Input: part model. Units: mm. Frame: model coordinates. A direction names the side the tool comes from. Coordinates: 2 decimals unless noted, no trailing zeros. Loops run counter-clockwise (first coordinate to the right, second up) from the corner with the lowest first, then second, coordinate; pieces in that order, holes last. Notation, with made-up numbers: (57, 67.25) -> (89, 67.25) arc R27 cw to (89, 87.25) -> close; hole circle Ø2 at (58, 77.5). An arc over 180 degrees is marked (long way). Put each result on its own line as item: value. Start each with the question number.
1) Cut plane B-B (z = -0.5). Return the cut outline in (x, y).
2) Cut plane A-A (z = 3). State how many separate pieces and enclosed holes the cut face has, plus the area to 3 significant figures.
3) Pull-direction query (X, two-part tool) for faces 1 (the flat face through (0, -2, 5.5)), 2 (the cylindrical face through (2.92, -14.18, 5.88)), 3 (the cylindrical face through (17.856, 3.771, 4.277)), 4 (the flat face through (0, 0, 6.5)); classes: pulls with the +X half, pulls with the -X half, needs draft (parallel to the pull), parting line crosses it, or undercut.
4) Set-up query: faces 5 (the cylindrical face through (1.269, 9.667, 2.712)), 6 (the cylindrical face through (8.19, 16.31, 4.28)), 7 (the cylindrical face through (1.03, -14.47, 5.48)). Return all of +Z, -Z, +X, -X, +Y, -Y with unobstructed straight access to the full face (end or side cutting, diameter ignored); none if empty.
5) Material intervals for L1, parallel to Y at x = 0, z = 1.1; L2, parallel to Z at x = -9, y = 1.5; L3, parallel to X at y = -4.5, z = 4, sorted ascending.
6) Contact query for flat-ended pins moving along their axis: P1, Ø8, axis at x = 7, y = 10, coming from the -Z side; P2, Ø4, axis at x = -3.5, z = 3, coming from the -Y side; P3, Ø4, axis at x = 13, z = 2.5, coming from the -Y side; P4, Ø6.5, axis at x = -1, y = 0, coming from the -Z side. Output: stop coordinate, or through.
from build123d import *

# Parameters (mm, degrees)
SKETCH_1_R               = 11
EXTRUDE_1_DEPTH          = 6.5
SKETCH_2_R               = 9.75
CUT_EXTRUDE_1_DEPTH      = 5.5
SKETCH_3_R               = 0.7
EXTRUDE_2_DEPTH          = 7.5
CHAMFER_1_SIZE           = 0.6
EXTRUDE_START            = -10
EXTRUDE_3_DEPTH          = 23
PATTERN_CIRCULAR_1_COUNT = 7
FILLET_1_R               = 0.3
SKETCH_5_OUTSIDE_W       = 86.532
SKETCH_5_OUTSIDE_H       = 84.877
SKETCH_5_OUTSIDE_R       = 18.25
CUT_EXTRUDE_2_DEPTH      = 23


with BuildPart() as part:
    # Sketch 1 → Extrude 1 (new body)
    with BuildSketch(Plane.XY):
        Circle(SKETCH_1_R)
    extrude(amount=EXTRUDE_1_DEPTH)

    # Sketch 2 → Cut-Extrude 1 (cut)
    with BuildSketch(Plane(origin=(0, 0, 0), x_dir=(-1, 0, 0), z_dir=(0, 0, -1))):
        Circle(SKETCH_2_R)
    extrude(amount=-CUT_EXTRUDE_1_DEPTH, mode=Mode.SUBTRACT)

    # Sketch 3 → Extrude 2 (add)
    with BuildSketch(Plane(origin=(0, 0, 5.5), x_dir=(-1, 0, 0), z_dir=(0, 0, -1))):
        Circle(SKETCH_3_R)
    extrude(amount=EXTRUDE_2_DEPTH)

    # Chamfer 1
    chamfer_1_edges = [part.edges().sort_by_distance(p)[0] for p in [
        (0.7, 0, -2),
    ]]
    chamfer(chamfer_1_edges, length=CHAMFER_1_SIZE)

    # Sketch 4 → Extrude 3 (add)
    with BuildSketch(Plane(origin=(0, 0, 0), x_dir=(1, 0, 0), z_dir=(0, 1, 0)).offset(EXTRUDE_START)):
        with BuildLine():
            ThreePointArc((3.75, -5.9), (2.910954768, -5.877455841), (2.076425924, -5.787640746))
            ThreePointArc((2.076425924, -5.787640746), (1.016898237, -5.476222818), (0.082906283, -4.886952865))
            ThreePointArc((0.082906283, -4.886952865), (-2.084101368, -2.63998988), (-3.75, 0))
            ThreePointArc((-3.75, 0), (-1.712075741, -2.552424329), (0.739315837, -4.710822941))
            ThreePointArc((0.739315837, -4.710822941), (2.002660979, -5.416468702), (3.40130611, -5.787640746))
            ThreePointArc((3.40130611, -5.787640746), (3.575082247, -5.845591808), (3.75, -5.9))
        make_face()
    extrude_3 = extrude(amount=-EXTRUDE_3_DEPTH)

    # Pattern Circular 1: Extrude 3 ×7 about axis
    pattern_circular_1_axis = Axis((0, 0, 0), (0, 0, 1))
    for i in range(1, PATTERN_CIRCULAR_1_COUNT):
        add(extrude_3.rotate(pattern_circular_1_axis, i * 360 / PATTERN_CIRCULAR_1_COUNT))

    # Fillet 1
    fillet_1_edges = [part.edges().sort_by_distance(p)[0] for p in [
        (-11, 0, 6.5),
    ]]
    fillet(fillet_1_edges, radius=FILLET_1_R)

    # Sketch 5 outside → Cut-Extrude 2 (cut)
    with BuildSketch(Plane.XY.offset(6.5)):
        with Locations((0, -0.8205)):
            Rectangle(SKETCH_5_OUTSIDE_W, SKETCH_5_OUTSIDE_H)
        Circle(SKETCH_5_OUTSIDE_R, mode=Mode.SUBTRACT)
    extrude(amount=-CUT_EXTRUDE_2_DEPTH, mode=Mode.SUBTRACT)


solid = part.part
Results found:
1. outline: circle Ø1.4 at (0, 0)
2. separate pieces: 2
2. enclosed holes: 1
2. area: 110 mm2
3. face 1: undercut
3. face 2: undercut
3. face 3: pulls with the +X half
3. face 4: needs draft
4. face 5: -Z
4. face 6: +Z, -Z, +X, +Y
4. face 7: +Z, -Y
5. L1: y = -11 to -9.75, -0.7 to 0.7, 9.75 to 11
5. L2: z = 5.5 to 6.5
5. L3: x = -10.04 to -8.65, 8.65 to 10.04
6. P1: stops at z = 0
6. P2: stops at y = -18.19
6. P3: stops at y = -13.79
6. P4: stops at z = -2
